Input: part model. Units: mm. Frame: model coordinates. A direction names the side the tool comes from. Coordinates: 2 decimals unless noted, no trailing zeros. Order: outer loops, then holes, each group sorted by start corner. A loop starts at its lowest first (then second) coordinate and runs counter-clockwise, first axis right, second up. Notation, with made-up numbers: (-21, 54) -> (29, 54) arc R19 ccw to (29, 69) -> close; hole circle Ø2 at (-19, -19). An arc over 180 degrees is marked (long way). Write each question's results on one line, items separated by ' | '.
```python
from build123d import *
from OCP.BRepFilletAPI import BRepFilletAPI_MakeFillet

# Parameters (mm, degrees)
SKETCH1_R           = 2.627
BOSS_EXTRUDE1_DEPTH = 6
BOSS_EXTRUDE2_START = -5.08
SKETCH1_3_W         = 38.1
SKETCH1_3_H         = 5.999999938
BOSS_EXTRUDE2_DEPTH = 25.4
SKETCH3_R           = 1.25
CUT_EXTRUDE1_DEPTH  = 45.654479015
FILLET1_R1          = 2.54
FILLET1_R2          = 5.08
SKETCH4_R           = 4.2145
SKETCH4_R_2         = 2.627
BOSS_EXTRUDE3_DEPTH = 2.54
BOSS_EXTRUDE4_START = 7.62
SKETCH4_2_R         = 4.2145
SKETCH4_2_R_2       = 2.627
BOSS_EXTRUDE4_DEPTH = 2.54
CHAMFER2_SIZE       = 2.54


with BuildPart() as part:
    # Sketch1 → Boss-Extrude1 (new body)
    with BuildSketch(Plane(origin=(5.08, 0, 0), x_dir=(0, 0, -1), z_dir=(1, 0, 0))):
        Polygon((-19.05, 0), (-19.05, -10.16), (0, -25.4), (19.05, -10.16), (19.05, 0), align=None)
        with Locations((0, -16.51)):
            Circle(SKETCH1_R, mode=Mode.SUBTRACT)
    boss_extrude1 = extrude(amount=BOSS_EXTRUDE1_DEPTH)

    # Sketch1<3> → Boss-Extrude2 (add)
    with BuildSketch(Plane(origin=(5.08, 0, 0), x_dir=(0, 0, -1), z_dir=(1, 0, 0)).offset(BOSS_EXTRUDE2_START)):
        with Locations((0, 2.999999969)):
            Rectangle(SKETCH1_3_W, SKETCH1_3_H)
    boss_extrude2 = extrude(amount=BOSS_EXTRUDE2_DEPTH)

    # Sketch3 → Cut-Extrude1 (cut, through all)
    with BuildSketch(Plane(origin=(0, 5.999999938, 0), x_dir=(1, 0, 0), z_dir=(0, 1, 0))):
        with Locations(Location((19.05, 12.7, 0), (0, 0, 270))):
            Circle(SKETCH3_R)
        with Locations(Location((19.05, -12.7, 0), (0, 0, 90))):
            Circle(SKETCH3_R)
    cut_extrude1 = extrude(amount=-CUT_EXTRUDE1_DEPTH, mode=Mode.SUBTRACT)

    # Mirror2: Boss-Extrude2, Cut-Extrude1 across plane
    add(boss_extrude2.mirror(Plane(origin=(0, 0, 0), x_dir=(0, 0, 1), z_dir=(1, 0, 0))))
    add(cut_extrude1.mirror(Plane(origin=(0, 0, 0), x_dir=(0, 0, 1), z_dir=(1, 0, 0))), mode=Mode.SUBTRACT)

    # Mirror3: Boss-Extrude1 across plane
    add(boss_extrude1.mirror(Plane(origin=(0, 0, 0), x_dir=(0, 0, 1), z_dir=(1, 0, 0))))

    # Fillet1: one fillet with a radius per group of edges: ONE call of the kernel's fillet builder (fillet() takes one radius for all edges)
    fillet1_edges_1 = [part.edges().sort_by_distance(p)[0] for p in [
        (8.08, -10.16, 19.05),
        (8.08, -10.16, -19.05),
        (11.08, 0, 0),
        (25.4, 2.999999969, 19.05),
        (25.4, 2.999999969, -19.05),
        (-25.4, 2.999999969, -19.05),
        (-25.4, 2.999999969, 19.05),
        (-8.08, -10.16, -19.05),
        (-8.08, -10.16, 19.05),
        (-5.08, 0, 0),
        (-11.08, 0, 0),
        (5.08, 0, 0),
    ]]
    fillet1_edges_2 = [part.edges().sort_by_distance(p)[0] for p in [
        (8.08, -25.4, 0),
        (-8.08, -25.4, 0),
    ]]
    fillet1 = BRepFilletAPI_MakeFillet(part.part.solid().wrapped)
    for e in fillet1_edges_1:
        fillet1.Add(FILLET1_R1, e.wrapped)
    for e in fillet1_edges_2:
        fillet1.Add(FILLET1_R2, e.wrapped)
    add(Compound.cast(fillet1.Shape()), mode=Mode.REPLACE)

    # Sketch4 → Boss-Extrude3 (add)
    with BuildSketch(Plane.ZY.offset(-5.08)):
        with Locations(Location((0, -16.51, 0), (0, 0, 180))):
            Circle(SKETCH4_R)
        with Locations((0, -16.51)):
            Circle(SKETCH4_R_2, mode=Mode.SUBTRACT)
    extrude(amount=BOSS_EXTRUDE3_DEPTH)

    # Sketch4<2> → Boss-Extrude4 (add)
    with BuildSketch(Plane.ZY.offset(-5.08).offset(BOSS_EXTRUDE4_START)):
        with Locations(Location((0, -16.51, 0), (0, 0, 180))):
            Circle(SKETCH4_2_R)
        with Locations((0, -16.51)):
            Circle(SKETCH4_2_R_2, mode=Mode.SUBTRACT)
    extrude(amount=BOSS_EXTRUDE4_DEPTH)

    # Chamfer2
    chamfer2_edges = [part.edges().sort_by_distance(p)[0] for p in [
        (5.08, -16.51, 4.2145),
        (-5.08, -16.51, 4.2145),
    ]]
    chamfer(chamfer2_edges, length=CHAMFER2_SIZE - 0.0001)  # a hair under: the kernel refuses the full size


solid = part.part
```
(1) Cut plane B-B, the plane x = 19.05. Return loops of the section in (y, z).
Return value:
outline: (0, -19.05) -> (6, -19.05) -> (6, -13.95) -> (0, -13.95) -> close; (0, -11.45) -> (6, -11.45) -> (6, 11.45) -> (0, 11.45) -> close; (0, 13.95) -> (6, 13.95) -> (6, 19.05) -> (0, 19.05) -> close
(2) Reachability of faces 4 (the face through (5.08, -8, 0)), 5 (the face through (-4.316, -0.724, 0.267)), 6 (the face through (11.08, -11, 0)), 7 (the face through (0, 0, 0)) from +Z, -Z, +X, -X, +Y, -Y: full face, straight path, thin tool, end or side. Return the list, or none.
Return value:
face 4: none | face 5: +Z, -Z | face 6: +Z, -Z, +X, -Y | face 7: +Z, -Z, -Y
(3) Pin query (flat end, axial travel): P1, Ø7, axis at y = -16.51, z = 0, coming from the +X side; P2, Ø6.5, axis at y = -12, z = 7.5, coming from the -X side; P3, Ø4, axis at x = 1, y = -15.5, coming from the +Z side. Return the tip coordinate at first contact, or that it passes through.
Return value:
P1: x = 11.08 | P2: x = -11.08 | P3: z = 4.6
(4) Cut plane A-A, the plane y = -3.25. Return loops of the section in (x, z).
Return value:
outline: (-11.08, -19.05) -> (-5.08, -19.05) -> (-5.08, 19.05) -> (-11.08, 19.05) -> close; (5.08, -19.05) -> (11.08, -19.05) -> (11.08, 19.05) -> (5.08, 19.05) -> close
(5) Line query: line 1 along X through (y, z) = (2.1, -12.7); line 2 along X through (y, z) = (-4, 8.5); line 3 along Y through (x, z) = (-9, 0). Output: solid intervals per line, ascending. Write a range as from..to.
Return value:
line 1: -25.4..-20.3, -17.8..17.8, 20.3..25.4 | line 2: -11.08..-5.08, 5.08..11.08 | line 3: -23.97..-19.14, -13.88..6
(6) Mould query, pull axis X, two halves, no side actions, for faces 1 (the face through (-24.636, 3.042, 18.326)), 2 (the face through (17.83, 3.04, -12.97)), 3 (the face through (-8.122, -10.025, 18.806)). Classes: +X half, -X half, draft (parallel to the pull), parting line (faces both ways), or undercut.
Return value:
face 1: -X half | face 2: undercut | face 3: draft
(7) Cut plane D-D, the plane z = -8.5. Return loops of the section in (x, y).
Return value:
outline: (-25.4, 0) -> (-13.62, 0) arc R2.54 cw to (-11.08, -2.54) -> (-11.08, -18.6) -> (-5.08, -18.6) -> (-5.08, -2.54) arc R2.54 cw to (-2.54, 0) -> (2.54, 0) arc R2.54 cw to (5.08, -2.54) -> (5.08, -18.6) -> (11.08, -18.6) -> (11.08, -2.54) arc R2.54 cw to (13.62, 0) -> (25.4, 0) -> (25.4, 6) -> (-25.4, 6) -> close
(8) Cut plane C-C, the plane z = 12.7. Return loops of the section in (x, y).
Return value:
outline: (-25.4, 0) -> (-20.3, 0) -> (-20.3, 6) -> (-25.4, 6) -> close; (-17.8, 0) -> (-13.62, 0) arc R2.54 cw to (-11.08, -2.54) -> (-11.08, -15.24) -> (-5.08, -15.24) -> (-5.08, -2.54) arc R2.54 cw to (-2.54, 0) -> (2.54, 0) arc R2.54 cw to (5.08, -2.54) -> (5.08, -15.24) -> (11.08, -15.24) -> (11.08, -2.54) arc R2.54 cw to (13.62, 0) -> (17.8, 0) -> (17.8, 6) -> (-17.8, 6) -> close; (20.3, 0) -> (25.4, 0) -> (25.4, 6) -> (20.3, 6) -> close
